from build123d import *

# Parameters (mm, degrees)
SKETCH1_R           = 31
SKETCH1_R_2         = 22
BOSS_EXTRUDE1_DEPTH = 40
BOSS_EXTRUDE2_START = 30
BOSS_EXTRUDE2_DEPTH = 10
BOSS_EXTRUDE3_START = 30
SKETCH1_4_R         = 22
SKETCH1_4_R_2       = 7.5
BOSS_EXTRUDE3_DEPTH = 20
BOSS_EXTRUDE4_DEPTH = 10
BOSS_EXTRUDE5_START = -10
SKETCH1_6_R         = 7.5
BOSS_EXTRUDE5_DEPTH = 20


with BuildPart() as part:
    # Sketch1 → Boss-Extrude1 (new body)
    # profile 1 of 2: a face of its own
    with BuildSketch(Plane(origin=(0, 0, 0), x_dir=(1, 0, 0), z_dir=(0, 1, 0))):
        with Locations(Location((0, 0, 0), (0, 0, 270))):
            Circle(SKETCH1_R)
        Circle(SKETCH1_R_2, mode=Mode.SUBTRACT)
    # profile 2 of 2: a face of its own
    with BuildSketch(Plane(origin=(0, 0, 0), x_dir=(1, 0, 0), z_dir=(0, 1, 0))):
        Circle(SKETCH1_R_2)
        with BuildLine():
            ThreePointArc((12.845232579, 2), (-13, 0), (12.845232579, -2))
            Line((12.845232579, -2), (17.845232579, -2))
            Line((17.845232579, -2), (17.845232579, 2))
            Line((17.845232579, 2), (12.845232579, 2))
        make_face(mode=Mode.SUBTRACT)
    extrude(amount=BOSS_EXTRUDE1_DEPTH)

    # Sketch1_3 → Boss-Extrude2 (add)
    with BuildSketch(Plane(origin=(0, 0, 0), x_dir=(1, 0, 0), z_dir=(0, 1, 0)).offset(BOSS_EXTRUDE2_START)):
        with BuildLine():
            Line((4.292307692, -30.701402161), (9.08353603, -30.031549164))
            Line((9.08353603, -30.031549164), (68.046153846, -21.788091856))
            ThreePointArc((68.046153846, -21.788091856), (43, 0), (68.046153846, 21.788091856))
            Line((68.046153846, 21.788091856), (4.292307692, 30.701402161))
            ThreePointArc((4.292307692, 30.701402161), (23.388688916, 20.346233823), (31, 0))
            ThreePointArc((31, 0), (23.388688916, -20.346233823), (4.292307692, -30.701402161))
        make_face()
    extrude(amount=BOSS_EXTRUDE2_DEPTH)

    # Sketch1_4 → Boss-Extrude3 (add)
    with BuildSketch(Plane(origin=(0, 0, 0), x_dir=(1, 0, 0), z_dir=(0, 1, 0)).offset(BOSS_EXTRUDE3_START)):
        with Locations(Location((65, 0, 0), (0, 0, 82.041168118))):
            Circle(SKETCH1_4_R)
        with Locations(Location((65, 0, 0), (0, 0, 270))):
            Circle(SKETCH1_4_R_2, mode=Mode.SUBTRACT)
    extrude(amount=BOSS_EXTRUDE3_DEPTH)

    # Sketch1_5 → Boss-Extrude4 (add)
    with BuildSketch(Plane(origin=(0, 0, 0), x_dir=(1, 0, 0), z_dir=(0, 1, 0))):
        with BuildLine():
            Line((-94.382971499, -79.823897994), (9.08353603, -30.031549164))
            Line((9.08353603, -30.031549164), (4.292307692, -30.701402161))
            ThreePointArc((4.292307692, -30.701402161), (-28.915707021, -11.175056488), (-17.469853837, 25.608674447))
            Line((-17.469853837, 25.608674447), (-116.321009242, -41.826102006))
            ThreePointArc((-116.321009242, -41.826102006), (-93.645771026, -40.54807031), (-81.923048454, -60))
            ThreePointArc((-81.923048454, -60), (-85.296700275, -71.70722655), (-94.382971499, -79.823897994))
        make_face()
    extrude(amount=BOSS_EXTRUDE4_DEPTH)

    # Sketch1_6 → Boss-Extrude5 (add)
    with BuildSketch(Plane(origin=(0, 0, 0), x_dir=(1, 0, 0), z_dir=(0, 1, 0)).offset(BOSS_EXTRUDE5_START)):
        with BuildLine():
            ThreePointArc((-116.321009242, -41.826102006), (-122.975607337, -71), (-94.382971499, -79.823897994))
            ThreePointArc((-94.382971499, -79.823897994), (-85.296700275, -71.70722655), (-81.923048454, -60))
            ThreePointArc((-81.923048454, -60), (-93.645771026, -40.54807031), (-116.321009242, -41.826102006))
        make_face()
        with Locations(Location((-103.923048454, -60, 0), (0, 0, 270))):
            Circle(SKETCH1_6_R, mode=Mode.SUBTRACT)
    extrude(amount=BOSS_EXTRUDE5_DEPTH)


solid = part.part
For this review, take the finished solid that the model builds, in its own axes (mm). A direction names the side the tool comes from. Coordinates: 2 decimals unless noted, no trailing zeros. Order: outer loops, then holes, each group sorted by start corner. A loop starts at its lowest first (then second) coordinate and runs counter-clockwise, first axis right, second up. Notation, with made-up numbers: (63.25, -11) - (86.25, -11) arc R18 ccw to (86.25, 5) - close; hole circle Ø1 at (29.5, 26). An arc over 180 degrees is marked (long way). Use one line per item in the form item = value.
Q1. Consider section D-D (x = 0). Give the boundary of the cut face in (y, z), then the cut area to 3 significant figures.
Checked values:
outline = (0, -31) - (40, -31) - (40, -13) - (0, -13) - close; (0, 13) - (40, 13) - (40, 31) - (10, 31) - (10, 34.4) - (0, 34.4) - close
area = 1,470 mm2
Q2. Consider section B-B (y = 32.5). Give the boundary of the cut face in (x, z), then the cut area to 3 significant figures.
Checked values:
outline = (4.29, -30.7) - (68.05, -21.79) arc R22 ccw to (68.05, 21.79) - (4.29, 30.7) arc R31 ccw (long way) to start; hole (12.85, -2) - (17.85, -2) - (17.85, 2) - (12.85, 2) arc R13 ccw (long way) to start; hole circle Ø15 at (65, 0)
area = 5,020 mm2
Q3. For probe 1 along X at (y, z) = (38, 0); probe 2 along Z at (x, y) = (0, 17); probe 3 along X at (y, z) = (18.5, 0), list the stretches that pass through material, from the lowest coordinate up. Write a range as from..to.
Checked values:
probe_1 = -31..-13, 17.85..57.5, 72.5..87
probe_2 = -31..-13, 13..31
probe_3 = -31..-13, 17.85..31
Q4. Draft analysis for pull direction X (two halves, no side actions). For faces 1 (the flat face through (18, 40, 6)), 2 (the flat face through (36.62, 34.93, -26.18)), 3 (the flat face through (15, 20, 2)), 4 (the flat face through (15, 20, -2)), state which applies: +X half, -X half, draft (parallel to the pull), parting line (faces both ways), or undercut.
Checked values:
face_1 = draft
face_2 = +X half
face_3 = undercut
face_4 = undercut
Q5. Consider section C-C (x = 70.5). Give the boundary of the cut face in (y, z), then the cut area to 3 significant figures.
Checked values:
outline = (30, -21.3) - (50, -21.3) - (50, -5.1) - (30, -5.1) - close; (30, 5.1) - (50, 5.1) - (50, 21.3) - (30, 21.3) - close
area = 648 mm2
Q6. For faces 5 (the flat face through (7.786, 4.93, 30.213)), 6 (the cylindrical face through (85.735, 42.082, -7.351)), 7 (the flat face through (17.845, 20, 0)), list the 3-axis set-ups (+Z, -Z, +X, -X, +Y, -Y) from which the entire face can be reached by the end or side of a thin tool; tool diameter is ignored.
Checked values:
face_5 = none
face_6 = +Y
face_7 = +Y, -Y
Q7. For P1, Ø3, axis at x = -62, z = 32, coming from the +Y side; P2, Ø5, axis at y = 17, z = -6.5, coming from the -X side; P3, Ø2.5, axis at x = 16, y = 18.5, coming from the +Z side, all flat-tipped, find the tip position at first contact; note any pin that passes through.
Checked values:
P1 = 10
P2 = -30.74
P3 = 27.27
Q8. Consider section A-A (z = 0). Give the boundary of the cut face in (x, y), then the cut area to 3 significant figures.
Checked values:
outline = (-55.01, 0) - (-13, 0) - (-13, 40) - (-31, 40) - (-31, 10) - (-55.01, 10) - close; (17.85, 0) - (31, 0) - (31, 30) - (57.5, 30) - (57.5, 50) - (43, 50) - (43, 40) - (17.85, 40) - close; (72.5, 30) - (87, 30) - (87, 50) - (72.5, 50) - close
area = 2,190 mm2
